Could you check a few things on this model? Use its own coordinates, in mm. Coordinates: 2 decimals unless noted, no trailing zeros. Loops run counter-clockwise (first coordinate to the right, second up) from the corner with the lowest first, then second, coordinate; pieces in that order, holes last. Notation, with made-up numbers: (11, 55) -> (59, 55) arc R14 ccw to (59, 65) -> close; hole circle Ø4 at (21, 37.5). An arc over 180 degrees is marked (long way). One line per question, with ' | ' between items.
Autodesk Inventor part; units mm, degrees
ref_plane "YZ Plane" through (0, 0, 0) normal (1, 0, 0) x (0, 1, 0)
ref_plane "XZ Plane" through (0, 0, 0) normal (0, 1, 0) x (-1, 0, 0)
ref_plane "XY Plane" through (0, 0, 0) normal (0, 0, 1) x (1, 0, 0)
sketch "Sketch1" plane through (0, 0, 0) normal (0, 0, 1) x (1, 0, 0)
  circle A0 centre (40, -0.1123) radius 1.75
  circle A1 centre (0, -0.1123) radius 1.75
  circle A2 centre (-40, -0.1123) radius 1.75
  line L0 (-44, 3.3877) -> (44, 3.3877)
  line L1 (-44, -3.3877) -> (-44, 3.3877)
  line L2 (44, -3.3877) -> (-44, -3.3877)
  line L3 (44, 3.3877) -> (44, -3.3877)
  circle A3 centre (-40, 64.7863) radius 1.75
  circle A4 centre (0, 64.7863) radius 1.75
  circle A5 centre (40, 64.7863) radius 1.75
  line L4 (44, 61.2863) -> (-44, 61.2863)
  line L5 (44, 68.0616) -> (44, 61.2863)
  line L6 (-44, 68.0616) -> (44, 68.0616)
  line L7 (-44, 61.2863) -> (-44, 68.0616)
  line L8 (44, 68.0616) -> (44, -3.3877)
  line L9 (44, -3.3877) -> (47, -3.3877)
  line L10 (47, 68.0616) -> (47, -3.3877)
  line L11 (44, 68.0616) -> (47, 68.0616)
  line L12 (-47, 68.0616) -> (-47, -3.3877)
  line L13 (-47, -3.3877) -> (-44, -3.3877)
  line L14 (-44, 68.0616) -> (-44, -3.3877)
  line L15 (-47, 68.0616) -> (-44, 68.0616)
  line L16 (-47, -3.3877) -> (-52, -3.3877)
  line L17 (-52, -3.3877) -> (-52, 68.0616)
  line L18 (-52, 68.0616) -> (-47, 68.0616)
  line L19 (-47, 68.0616) -> (-47, -3.3877)
  line L20 (47, -3.3877) -> (52, -3.3877)
  line L21 (52, -3.3877) -> (52, 68.0616)
  line L22 (52, 68.0616) -> (47, 68.0616)
  line L23 (47, 68.0616) -> (47, -3.3877)
  point P0 (0, 0)
  dimension "d0" = 5
  dimension "d1" = 5
extrude "Extrusion1" add sketch "Sketch1" along normal blind 3
equation "\"BendRadius\" = Thickness"
equation "\"BendReliefWidth\" = Thickness"
equation "\"BendReliefDepth\" = 0.5 * Thickness"
equation "\"CornerReliefSize\" = 4 * Thickness"
equation "\"MinimumRemnant\" = 2 * Thickness"
equation "\"TransitionRadius\" = BendRadius"
equation "\"JacobiRadiusSize\" = Thickness"
equation "\"GapSize\" = Thickness"
properties part number "КВ33.000.104 - Крышка" material "ABS Plastic"
1) I need wall thicknesses on line 1 along Y through (x, z) = (-40, 0.8). Which ranges of the line are inside material? Lowest first, please. Write a range as from..to.
Data:
line 1: -3.39..-1.86, 1.64..63.04, 66.54..68.06
2) I'm going to push a flat-ended pin straight in: pin 1 Ø2 at (x, y) = (0, -0.11) entering from -Z. Where does the tip first touch, or does it pass through?
Data:
pin 1: through
3) If we section it at A-A on x = 40: Please give me the cut outline in (y, z).
Data:
outline: (-3.39, 0) -> (-1.86, 0) -> (-1.86, 3) -> (-3.39, 3) -> close; (1.64, 0) -> (63.04, 0) -> (63.04, 3) -> (1.64, 3) -> close; (66.54, 0) -> (68.06, 0) -> (68.06, 3) -> (66.54, 3) -> close
4) We'd pull the mould along X, two halves only. Please class faces 1 (the face through (52, 32, 1)), 2 (the face through (-38.4, 0.6, 1.5)), 3 (the face through (-1, -3.388, 1)): pulls with the +X half, pulls with the -X half, needs draft (parallel to the pull), parting line crosses it, or undercut.
Data:
face 1: pulls with the +X half | face 2: undercut | face 3: needs draft
